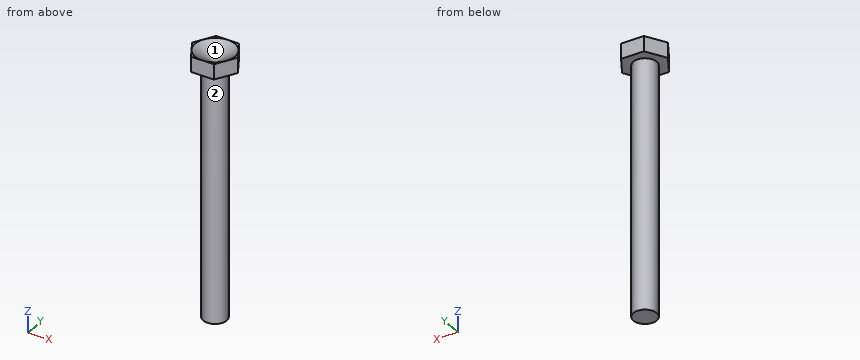
```python
from build123d import *

# Parameters (mm, degrees)
SKETCH1_R           = 10
BOSS_EXTRUDE1_DEPTH = 110
BOSS_EXTRUDE2_DEPTH = 6.5


with BuildPart() as part:
    # Sketch1 → Boss-Extrude1 (new, symmetric)
    with BuildSketch(Plane.XY):
        Circle(SKETCH1_R)
    extrude(amount=BOSS_EXTRUDE1_DEPTH, both=True)

    # Sketch3 → Boss-Extrude2 (add, symmetric)
    with BuildSketch(Plane.XY.offset(110)):
        Polygon((19.629909152, 0), (9.814954576, 17), (-9.814954576, 17), (-19.629909152, 0), (-9.814954576, -17), (9.814954576, -17), align=None)
    extrude(amount=BOSS_EXTRUDE2_DEPTH, both=True)

    # Cut-Extrude1 cone 1 section (through the dimple's axis) → Cut-Extrude1 (revolve, cut)
    with BuildSketch(Plane(origin=(0, 0, 116.5), x_dir=(0, -1, 0), z_dir=(1, 0, 0))):
        Polygon((0, 0), (17, 0), (0, 9.814954576), align=None)
    revolve(axis=Axis((0, 0, 116.5), (0, 0, -1)), mode=Mode.SUBTRACT)


solid = part.part
```
Input: part model. Units: mm. Frame: model coordinates. Face numbers are marked on the shaded views. Give positions to 0.01 mm unless a question says otherwise; leave off trailing zeros. Order: outer loops, then holes, each group sorted by start corner. A loop starts at its lowest first (then second) coordinate and runs counter-clockwise, first axis right, second up. Notation, with made-up numbers: (54.25, -8.75) - (65.25, -8.75) arc R25 ccw to (65.25, 8.25) - close; hole circle Ø4 at (64.25, -18.5). An arc over 180 degrees is marked (long way). Put each result on its own line as item: value.
Item 1: Section query A-A, the plane z = 77.5. Return loops of the section in (x, y), then the cut area to 3 significant figures.
Found:
outline: circle Ø20 at (0, 0)
area: 314 mm^2
Item 2: Draft query along X for the marked faces 1 and 2. Return one class per face: +X half, -X half, draft (parallel to the pull), parting line (faces both ways), or undercut.
Found:
face 1: undercut
face 2: parting line
Item 3: Contact query for flat-ended pins moving along their axis: pin 1 (1.5 mm diameter, centred on x = 8, y = 0.5, fed in from +Z); pin 2 (8 mm diameter, centred on x = -3, z = -68, fed in from +Y); pin 3 (6 mm diameter, centred on x = 9.5, z = 1, fed in from -Y); pin 4 (5 mm diameter, centred on x = -5, y = 10.5, fed in from -Z). Output: stop coordinate, or through.
Found:
pin 1: stops at z = 111.75
pin 2: stops at y = 10
pin 3: stops at y = -7.6
pin 4: stops at z = -110
Item 4: Ray query, L1, parallel to Z at x = -18, y = 1; L2, parallel to X at y = 0.5, z = -21; L3, parallel to Y at x = -2, z = 54. Return the intervals inside material, ascending. Write a range as from..to.
Found:
L1: z = 103.5..116.5
L2: x = -9.99..9.99
L3: y = -9.8..9.8
